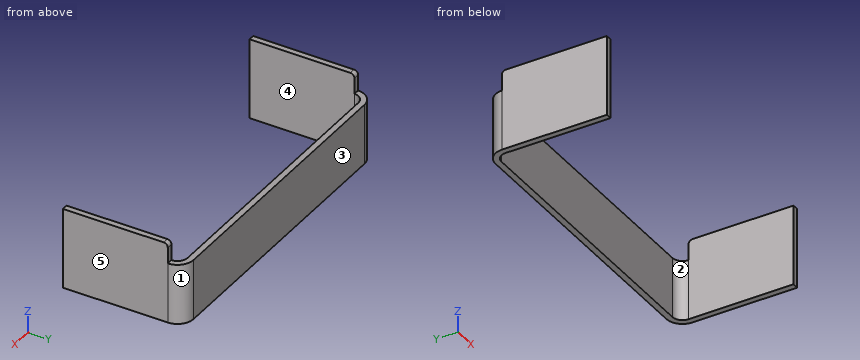
Autodesk Inventor part; units mm, degrees
ref_plane "YZ Plane" through (0, 0, 0) normal (1, 0, 0) x (0, 1, 0)
ref_plane "XZ Plane" through (0, 0, 0) normal (0, 1, 0) x (-1, 0, 0)
ref_plane "XY Plane" through (0, 0, 0) normal (0, 0, 1) x (1, 0, 0)
sketch "Sketch1" plane through (0, 0, 0) normal (0, 1, 0) x (-1, 0, 0)
  line L0 (78, 15) -> (-78, 15)
  line L1 (-78, 15) -> (-78, -15)
  line L2 (-78, -15) -> (78, -15)
  line L3 (78, -15) -> (78, 15)
  line L4 (78, 15) -> (-78, -15) construction
  line L5 (-78, 15) -> (78, -15) construction
  point P0 (0, 0)
  dimension "d37" = 156
  dimension "d38" = 30
extrude "Plate1" add sketch "Sketch1" along normal blind 3
sketch "Sketch4" plane through (-75, 3, -15) normal (-1, 0, 0) x (0, -1, 0)
  line L0 (0, 30) -> (0, 0)
  line L1 (0, 0) -> (60, 0)
  line L2 (60, 0) -> (60, 30)
  line L3 (60, 30) -> (0, 30)
edge flange "Flange1" height 60 angle 90 thickness 3 bend radius 5 thickness toward (-1, 0, 0) relief round relief width 3 relief depth 1.5 corner gap 5 corner form 0 edges at (-78, 0, 0) (78, 0, 0) wall of the first edge with corners at (-75, 3, 15) (-75, 3, -15) (-75, -57, -15) (-75, -57, 15)
bend "Bend1"
corner "Corner1"
sketch "Sketch5" plane through (-78, -57, 15) normal (0, 0, 1) x (1, 0, 0)
  line L0 (3, 52) -> (0, 52)
  line L1 (0, 52) -> (0, 0)
  line L2 (3, 0) -> (0, 0)
  line L3 (3, 52) -> (3, 0)
  point P0 (78, 57)
extrude "Extrusion2" add sketch "Sketch5" along normal blind 10
mirror "Mirror1" about plane through (0, 0, 0) normal (1, 0, 0) of "Extrusion2"
fillet "Fillet1" radius 2 2 edges at (76.5, -5, 25) (-76.5, -5, 25)
equation "\"d6\" = Thickness"
equation "\"d39\" = BendReliefWidth"
equation "\"d40\" = BendReliefDepth"
equation "\"d41\" = MinimumRemnant"
equation "\"d42\" = TransitionRadius"
equation "\"d45\" = BendRadius"
equation "\"d46\" = CornerReliefSize"
equation "\"d47\" = GapSize"
equation "\"d48\" = JacobiRadiusSize"
equation "\"BendReliefWidth\" = Thickness"
equation "\"BendReliefDepth\" = 0.5 * Thickness"
equation "\"CornerReliefSize\" = 4 * Thickness"
equation "\"MinimumRemnant\" = 2 * Thickness"
equation "\"TransitionRadius\" = BendRadius"
equation "\"JacobiRadiusSize\" = BendRadius"
equation "\"GapSize\" = Thickness"
properties part number "MSC 923 step" material "Stainless Steel"
Can you work these out from the model? Positions are in its coordinate system, mm. Face numbers are marked on the shaded views. A direction names the side the tool comes from. Give positions to 0.01 mm unless a question says otherwise; leave off trailing zeros. Write each loop counter-clockwise with the first axis right and the second up, starting at its lowest first coordinate (ties: lowest second). Pieces come first, ordered by that corner, then holes. Notation, with made-up numbers: (25, 60.25) - (47, 60.25) arc R17 cw to (47, 73.25) - close; hole circle Ø11 at (3, -24). An arc over 180 degrees is marked (long way). Write item = value, one per line. Start each with the question number.
1. On a 3-axis mill with a long thin cutter (end or side, diameter ignored), from which of +Z, -Z, +X, -X, +Y, -Y can I reach the whole of each face in a straight line? I mean the marked faces 4 and 5. Say none if no direction works.
2. Imagine slicing it at A-A (y = -26.5). Please give me the cut outline in (x, z).
3. For pin 1 (1.5 mm diameter, centred on x = -76.5, z = 19.5, fed in from +Y); pin 2 (2 mm diameter, centred on x = -4, z = 12.5, fed in from -Y); pin 3 (6.5 mm diameter, centred on x = 1, y = -0.5, fed in from +Z), each with a flat end and sliding along its axis, tell me the tip position at first contact or that it passes through.
4. Imagine slicing it at B-B (z = -4.5). Please give me the cut outline in (x, y), and give its area (3 significant figures).
5. Please list where these lines run through material, in increasing order: line 1 (X direction, y = -39, z = 5); line 2 (Y direction, x = -55, z = 7.5); line 3 (X direction, y = -3, z = -5.5).
6. Imagine slicing it at C-C (y = -2). Please give me the cut outline in (x, z), and give its area (3 significant figures).
7. Imagine slicing it at D-D (x = 52.5). Please give me the cut outline in (y, z), and give its area (3 significant figures).
8. Thinking about a two-plate mould opening in X: for the marked faces 1, 2 and 3, which applies, released by +X, released by -X, zero draft, split by the parting line, or undercut?
Worked answers:
q1.face_4 = +Z, -Z, -Y
q1.face_5 = +Z, -Z, +X, +Y, -Y
q2.outline = (-78, -15) - (-75, -15) - (-75, 25) - (-78, 25) - close; (75, -15) - (78, -15) - (78, 25) - (75, 25) - close
q3.pin_1 = -5
q3.pin_2 = 0
q3.pin_3 = 15
q4.outline = (-78, -57) - (-75, -57) - (-75, -5) arc R5 cw to (-70, 0) - (70, 0) arc R5 cw to (75, -5) - (75, -57) - (78, -57) - (78, -5) arc R8 ccw to (70, 3) - (-70, 3) arc R8 ccw to (-78, -5) - close
q4.area = 793 mm2
q5.line_1 = -78 to -75, 75 to 78
q5.line_2 = 0 to 3
q5.line_3 = -77.75 to -74.58, 74.58 to 77.75
q6.outline = (-77.42, -15) - (-74, -15) - (-74, 15) - (-77.42, 15) - close; (74, -15) - (77.42, -15) - (77.42, 15) - (74, 15) - close
q6.area = 205 mm2
q7.outline = (0, -15) - (3, -15) - (3, 15) - (0, 15) - close
q7.area = 90.0 mm2
q8.face_1 = released by +X
q8.face_2 = undercut
q8.face_3 = zero draft
